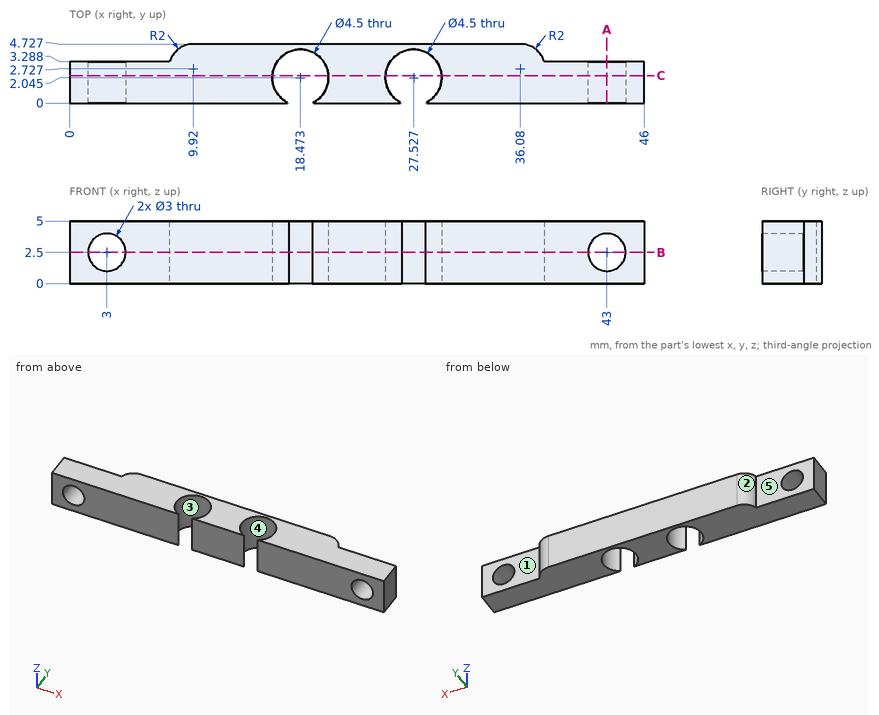
Can you work these out from the drawing? Everything is in mm from the part's minimum corner. A direction names the side the tool comes from. Coordinates: 2 decimals unless noted, no trailing zeros. Loops run counter-clockwise (first coordinate to the right, second up) from the corner with the lowest first, then second, coordinate; pieces in that order, holes last.
1. Imagine slicing it at A-A, the plane x = 43. Please give me the cut outline in (y, z).
2. If we mould it in two halves opening along X, with no side actions, what happens to the marked faces 1, 2 and 3? For each: pulls with the +X half, pulls with the -X half, needs draft (parallel to the pull), parting line crosses it, or undercut.
3. For P1, Ø1.5, axis at x = 9, z = 3.5, coming from the +Y side; P2, Ø2.5, axis at x = 27.53, y = 2.05, coming from the -Z side, each with a flat end and sliding along its axis, tell me the tip position at first contact or that it passes through.
4. Imagine slicing it at B-B, the plane z = 2.5. Count the separate pieces of the cut face and the enclosed holes in it, and give its area (3 significant figures).
5. I need wall thicknesses on L1, parallel to X at y = 2.25, z = 4.7; L2, parallel to Z at x = 3, y = 1.1; L3, parallel to X at y = 3.95, z = 3.35 (1 decimal). Which ranges of each line are inside material? Lowest first, please.
6. For the marked faces 4 and 5, which set-ups out of +Z, -Z, +X, -X, +Y, -Y let a thin tool reach every point of the face, with its end or its side?
7. Imagine slicing it at C-C, the plane y = 2.2. Please give me the cut outline in (x, z), and give its area (3 significant figures).
Taken from the geometry:
1. outline: (0, 0) - (3.29, 0) - (3.29, 1) - (0, 1) - close; (0, 4) - (3.29, 4) - (3.29, 5) - (0, 5) - close
2. face 1: needs draft
2. face 2: pulls with the -X half
2. face 3: undercut
3. P1: stops at y = 4.72
3. P2: passes through
4. separate pieces: 3
4. enclosed holes: 0
4. area: 142 mm2
5. L1: x = 0 to 16.23, 20.71 to 25.29, 29.77 to 46
5. L2: z = 0 to 1, 4 to 5
5. L3: x = 8.3 to 17.3, 19.7 to 26.3, 28.7 to 37.7
6. face 4: +Z, -Z
6. face 5: +Z, -Z, -X, +Y
7. outline: (0, 0) - (16.23, 0) - (16.23, 5) - (0, 5) - close; (20.72, 0) - (25.28, 0) - (25.28, 5) - (20.72, 5) - close; (29.77, 0) - (46, 0) - (46, 5) - (29.77, 5) - close; hole circle Ø3 at (3, 2.5); hole circle Ø3 at (43, 2.5)
7. area: 171 mm2
